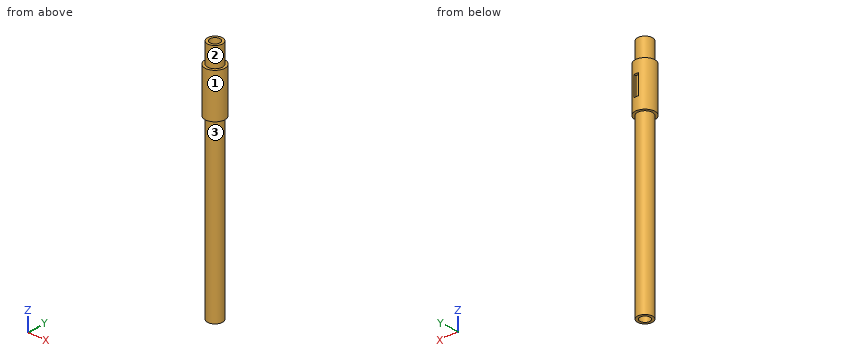
```python
from build123d import *

# Parameters (mm, degrees)
SKETCH1_R           = 12.7
SKETCH1_R_2         = 6.35
BOSS_EXTRUDE1_DEPTH = 304.8
SKETCH3_R           = 19.05
SKETCH3_R_2         = 9.525
CUT_EXTRUDE2_DEPTH  = 254
CUT_EXTRUDE3_DEPTH  = 25.4
CUT_EXTRUDE5_START  = -25.4
SKETCH2_R           = 19.05
SKETCH2_R_2         = 9.525
CUT_EXTRUDE5_DEPTH  = 25.4


with BuildPart() as part:
    # Sketch1 → Boss-Extrude1 (new body)
    with BuildSketch(Plane.XY):
        Circle(SKETCH1_R)
        Circle(SKETCH1_R_2, mode=Mode.SUBTRACT)
    extrude(amount=-BOSS_EXTRUDE1_DEPTH)

    # Sketch3 → Cut-Extrude2 (cut)
    with BuildSketch(Plane.XY.offset(-81.788)):
        Circle(SKETCH3_R)
        Circle(SKETCH3_R_2, mode=Mode.SUBTRACT)
    extrude(amount=-CUT_EXTRUDE2_DEPTH, mode=Mode.SUBTRACT)

    # Sketch4 → Cut-Extrude3 (cut)
    with BuildSketch(Plane.XY.offset(-40.894)):
        Polygon((-3.175, 12.296722124), (-3.175, 15.852722124), (3.175, 15.852722124), (3.175, 12.296722124), (3.175, 9.502722124), (-3.175, 9.502722124), align=None)
    extrude(amount=-CUT_EXTRUDE3_DEPTH, mode=Mode.SUBTRACT)

    # Sketch2 → Cut-Extrude5 (cut)
    with BuildSketch(Plane.XY.offset(CUT_EXTRUDE5_START)):
        Circle(SKETCH2_R)
        Circle(SKETCH2_R_2, mode=Mode.SUBTRACT)
    extrude(amount=CUT_EXTRUDE5_DEPTH, mode=Mode.SUBTRACT)


solid = part.part
```
Check sheet for the modelled part. Datum: model origin and axes. Units: mm. Face numbers are marked on the shaded views. A direction names the side the tool comes from. Coordinates: 2 decimals unless noted, no trailing zeros. Loops run counter-clockwise (first coordinate to the right, second up) from the corner with the lowest first, then second, coordinate; pieces in that order, holes last. Notation, with made-up numbers: M 88,1 L 103,1 A15 ccw 103,8 Z; hole C 71.5,71.25 d8. An arc over 180 degrees is marked long. Answer as a JSON object with one key per item and string values.
1. Sectioned sample at D-D on z = -162. Record the cut outline in (x, y) (3 decimals), and give its area (3 significant figures).
Outcome:
{"outline": "C 0,0 d19.05; hole C 0,0 d12.7", "area": "158 mm²"}
2. Sectioned sample at C-C on z = -47.5. Record the cut outline in (x, y) (3 decimals), and give its area (3 significant figures).
Outcome:
{"outline": "M -3.175,9.503 L -3.175,12.297 A12.7 ccw long 3.175,12.297 L 3.175,9.503 Z; hole C 0,0 d12.7", "area": "361 mm²"}
3. Depth check by flat-ended pin: P1, Ø0.8, axis at y = 11, z = -52, coming from the +X side (3 decimals); P2, Ø3, axis at y = 2, z = -55, coming from the -X side; P3, Ø5, axis at x = -1.5, y = 0, coming from the +Z side; P4, Ø5, axis at x = -8, y = -4, coming from the +Z side. Enter the tip coordinate at first touch or a pass-through.
Outcome:
{"P1": "x = 6.995", "P2": "x = -12.69", "P3": "through", "P4": "z = 0"}
4. Sectioned sample at B-B on y = 0. Record the cut outline in (x, z) (3 decimals).
Outcome:
{"outline": "M -12.7,-81.788 L -9.525,-81.788 L -9.525,-304.8 L -6.35,-304.8 L -6.35,0 L -9.525,0 L -9.525,-25.4 L -12.7,-25.4 Z; M 6.35,-304.8 L 9.525,-304.8 L 9.525,-81.788 L 12.7,-81.788 L 12.7,-25.4 L 9.525,-25.4 L 9.525,0 L 6.35,0 Z"}
5. Scan lines: L1, parallel to Y at x = 0, z = -121.5 (3 decimals); L2, parallel to X at y = 0.75, z = -240; L3, parallel to X at y = 3.75, z = -291.5. Record each from-to range of solid material in increasing order. Write a range as from..to.
Outcome:
{"L1": "-9.525..-6.35, 6.35..9.525", "L2": "-9.5..-6.31, 6.31..9.5", "L3": "-8.76..-5.12, 5.12..8.76"}
6. Sectioned sample at A-A on x = 0. Record the cut outline in (y, z) (3 decimals).
Outcome:
{"outline": "M -12.7,-81.788 L -9.525,-81.788 L -9.525,-304.8 L -6.35,-304.8 L -6.35,0 L -9.525,0 L -9.525,-25.4 L -12.7,-25.4 Z; M 6.35,-304.8 L 9.525,-304.8 L 9.525,-81.788 L 12.7,-81.788 L 12.7,-66.294 L 9.503,-66.294 L 9.503,-40.894 L 12.7,-40.894 L 12.7,-25.4 L 9.525,-25.4 L 9.525,0 L 6.35,0 Z"}
7. Access from +Z, -Z, +X, -X, +Y, -Y to the whole of each face (thin tool, end or side, straight path). Record for the marked faces 1, 2 and 3.
Outcome:
{"face 1": "+Z, -Z", "face 2": "+Z", "face 3": "-Z"}
